Autodesk Inventor part; units mm, degrees
ref_plane "YZ Plane" through (0, 0, 0) normal (1, 0, 0) x (0, 1, 0)
ref_plane "XZ Plane" through (0, 0, 0) normal (0, 1, 0) x (-1, 0, 0)
ref_plane "XY Plane" through (0, 0, 0) normal (0, 0, 1) x (1, 0, 0)
sketch "Sketch1" plane through (0, 0, 0) normal (0, 1, 0) x (-1, 0, 0)
  line L0 (0, 0) -> (50, 0)
  line L1 (50, 0) -> (50, -35)
  line L2 (50, -35) -> (0, -35)
  line L3 (0, -35) -> (0, 0)
  dimension "d0" = 50
  dimension "d1" = 35
extrude "Extrusion1" add sketch "Sketch1" along normal blind 10
sketch "Sketch2" plane through (0, 10, 0) normal (0, 1, 0) x (1, 0, 0)
  circle A0 centre (-25, 17.5) radius 11.25
  line L0 (0, 35) -> (-50, 35)
  line L1 (-50, 35) -> (-50, 0)
  point P0 (0, 0)
  dimension "d4" = 22.5
  dimension "d5" = 17.5
  dimension "d6" = 25
extrude "Extrusion2" cut sketch "Sketch2" against normal blind 5
sketch "Sketch3" plane through (0, 10, 0) normal (0, 1, 0) x (1, 0, 0)
  line L0 (-50, 35) -> (-50, 0)
  line L1 (-50, 0) -> (0, 0)
  line L2 (0, 0) -> (0, 35)
  line L3 (0, 35) -> (-50, 35)
  point P0 (-43.5, 8)
  point P1 (-6.5, 27)
  dimension "d9" = 6.5
  dimension "d10" = 8
  dimension "d11" = 6.5
  dimension "d12" = 8
hole "Hole1" at (-43.5, 10, -8) at (-6.5, 10, -27) direction (0, -1, 0) diameter 4.5 depth 20 tip angle 118 counterbore diameter 8.5 counterbore depth 4
fillet "Fillet1" radius 4 1 edges at (0, 5, 0)
fillet "Fillet2" radius 4 3 edges at (0, 5, -35) (-50, 5, -35) (-50, 5, 0)
properties part number "Small Bracket (LHS)"
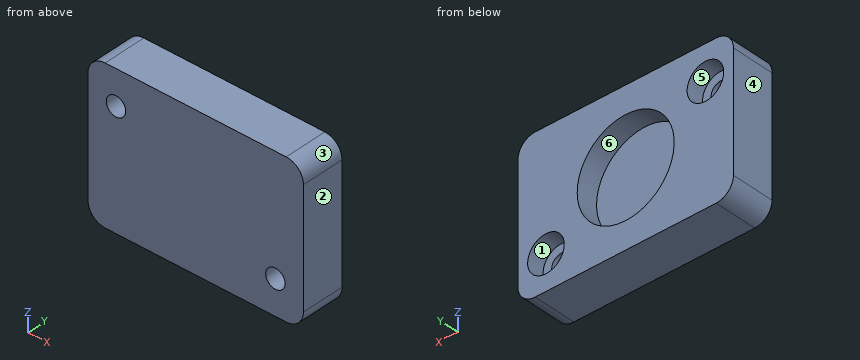
Model file for the job. Use its own axes, mm. Face numbers are marked on the shaded views. A direction names the side the tool comes from. Give positions to 0.01 mm unless a question says otherwise; leave off trailing zeros. Write each loop counter-clockwise with the first axis right and the second up, starting at its lowest first coordinate (ties: lowest second). Pieces come first, ordered by that corner, then holes. Notation, with made-up numbers: M -30,-1 L 0,-1 A22 cw 0,33 Z; hole C -23,-28.75 d10. An arc over 180 degrees is marked long. Use a Markdown table: item, result.
1) Pin check, flat tips, straight feed: pin 1 (2.5 mm diameter, centred on x = -5.5, z = -26.5, fed in from +Y); pin 2 (4 mm diameter, centred on x = -43.5, z = -8, fed in from +Y). Stop position of each tip, or through.
Responses:
| item | result |
|---|---|
| pin 1 | stops at y = 6 |
| pin 2 | passes through |
2) Cut at C-C (z = -17.5). List the corners of the cut face in (x, y).
Responses:
| item | result |
|---|---|
| outline | M -50,0 L 0,0 L 0,10 L -13.75,10 L -13.75,5 L -36.25,5 L -36.25,10 L -50,10 Z |
3) Cut at D-D (y = 3.25). List the corners of the cut face in (x, z), and give its area (3 significant figures).
Responses:
| item | result |
|---|---|
| outline | M -50,-31 A4 ccw -46,-35 L -4,-35 A4 ccw 0,-31 L 0,-4 A4 ccw -4,0 L -46,0 A4 ccw -50,-4 Z; hole C -43.5,-8 d4.5; hole C -6.5,-27 d4.5 |
| area | 1,700 mm2 |
4) Drill centre lines: line 1 (Z direction, x = -43.5, y = 7.95); line 2 (X direction, y = 7.85, z = -17.5); line 3 (Z direction, x = -6.5, y = 3.9). Where is each one in solid material? Low to high. Write a range as from..to.
Responses:
| item | result |
|---|---|
| line 1 | z = -35..-12.25, -3.75..0 |
| line 2 | x = -50..-36.25, -13.75..0 |
| line 3 | z = -35..-29.25, -24.75..0 |
5) Cut at B-B (z = -8). List the corners of the cut face in (x, y), and give its area (3 significant figures).
Responses:
| item | result |
|---|---|
| outline | M -50,0 L -45.75,0 L -45.75,6 L -47.75,6 L -47.75,10 L -50,10 Z; M -41.25,0 L 0,0 L 0,10 L -18.97,10 L -18.97,5 L -31.03,5 L -31.03,10 L -39.25,10 L -39.25,6 L -41.25,6 Z |
| area | 379 mm2 |
6) Pull direction Z, two halves, no side cores. Call the marked faces 3, 4, 5 and 6: +Z half, -Z half, draft (parallel to the pull), parting line (faces both ways), or undercut.
Responses:
| item | result |
|---|---|
| face 3 | +Z half |
| face 4 | draft |
| face 5 | undercut |
| face 6 | undercut |
7) Cut at A-A (y = 8.25). List the corners of the cut face in (x, z), and give its area (3 significant figures).
Responses:
| item | result |
|---|---|
| outline | M -50,-31 A4 ccw -46,-35 L -4,-35 A4 ccw 0,-31 L 0,-4 A4 ccw -4,0 L -46,0 A4 ccw -50,-4 Z; hole C -43.5,-8 d8.5; hole C -25,-17.5 d22.5; hole C -6.5,-27 d8.5 |
| area | 1,230 mm2 |
8) Tool access for the marked faces 1 and 2: list every direction of +Z, -Z, +X, -X, +Y, -Y with a clear straight run to the whole face (end or side of a thin tool).
Responses:
| item | result |
|---|---|
| face 1 | +Y |
| face 2 | +Z, -Z, +X, +Y, -Y |
